```python
from build123d import *

# Parameters (mm, degrees)
SKETCH1_R               = 11.7
BOSS_EXTRUDE1_DEPTH     = 35
SKETCH2_R               = 10
BOSS_EXTRUDE3_DEPTH     = 51.8
SKETCH3_R               = 3
CUT_EXTRUDE1_DEPTH      = 90.32860684
CUT_EXTRUDE1_DEPTH_BACK = 90.32860684
SKETCH6_W               = 28.4
SKETCH6_H               = 118.8
CUT_EXTRUDE3_DEPTH      = 75.564871086
SKETCH8_R               = 10
SKETCH8_R_2             = 3
CUT_EXTRUDE4_DEPTH      = 5
SKETCH7_R               = 4
SKETCH7_R_2             = 3
BOSS_EXTRUDE4_DEPTH     = 5
FILLET1_R               = 10


with BuildPart() as part:
    # Sketch1 → Boss-Extrude1 (new body)
    with BuildSketch(Plane(origin=(0, 0, 0), x_dir=(0, 0, -1), z_dir=(1, 0, 0))):
        Polygon((-28.4, -59.4), (-23.4, -59.4), (-23.4, -14.4), (23.4, -14.4), (23.4, -59.4), (28.4, -59.4), (28.4, 59.4), (-28.4, 59.4), align=None)
        with Locations((0, 24)):
            Circle(SKETCH1_R, mode=Mode.SUBTRACT)
    extrude(amount=BOSS_EXTRUDE1_DEPTH)

    # Sketch2 → Boss-Extrude3 (add)
    with BuildSketch(Plane.XY.offset(28.4)):
        with Locations(Location((17.5, -34.4, 0), (0, 0, 90))):
            Circle(SKETCH2_R)
        with BuildLine():
            Line((0, -24.717541634), (0, -13.4))
            Line((0, -13.4), (35, -13.4))
            Line((35, -13.4), (35, -24.717541634))
            ThreePointArc((35, -24.717541634), (17.5, -14.4), (0, -24.717541634))
        make_face()
    extrude(amount=-BOSS_EXTRUDE3_DEPTH)

    # Sketch3 → Cut-Extrude1 (cut, two sides)
    with BuildSketch(Plane.XY.offset(28.4)) as cut_extrude1_sk:
        with Locations((10.25, 49.4)):
            Circle(SKETCH3_R)
        with Locations((17.5, -34.4)):
            Circle(SKETCH3_R)
        with Locations((10.25, 2.3)):
            Circle(SKETCH3_R)
        with Locations((24.75, 2.3)):
            Circle(SKETCH3_R)
        with Locations((24.75, 49.4)):
            Circle(SKETCH3_R)
    extrude(amount=CUT_EXTRUDE1_DEPTH, mode=Mode.SUBTRACT)
    extrude(cut_extrude1_sk.sketch, amount=-CUT_EXTRUDE1_DEPTH_BACK, mode=Mode.SUBTRACT)

    # Sketch6 → Cut-Extrude3 (cut, through all)
    with BuildSketch(Plane(origin=(35, 0, 0), x_dir=(0, 0, -1), z_dir=(1, 0, 0))):
        with Locations((14.2, 0)):
            Rectangle(SKETCH6_W, SKETCH6_H)
    extrude(amount=-CUT_EXTRUDE3_DEPTH, mode=Mode.SUBTRACT)

    # Sketch8 → Cut-Extrude4 (cut)
    with BuildSketch(Plane(origin=(0, 0, 0), x_dir=(-1, 0, 0), z_dir=(0, 0, -1))):
        with Locations(Location((-17.5, -34.4, 0), (0, 0, 270))):
            Circle(SKETCH8_R)
        with Locations(Location((-17.5, -34.4, 0), (0, 0, 180))):
            Circle(SKETCH8_R_2, mode=Mode.SUBTRACT)
    extrude(amount=-CUT_EXTRUDE4_DEPTH, mode=Mode.SUBTRACT)

    # Sketch7 → Boss-Extrude4 (add)
    with BuildSketch(Plane(origin=(0, 0, 0), x_dir=(-1, 0, 0), z_dir=(0, 0, -1))):
        with Locations(Location((-24.75, 49.4, 0), (0, 0, 270))):
            Circle(SKETCH7_R)
        with Locations(Location((-24.75, 49.4, 0), (0, 0, 180))):
            Circle(SKETCH7_R_2, mode=Mode.SUBTRACT)
        with Locations(Location((-10.25, 49.4, 0), (0, 0, 270))):
            Circle(SKETCH7_R)
        with Locations(Location((-10.25, 49.4, 0), (0, 0, 180))):
            Circle(SKETCH7_R_2, mode=Mode.SUBTRACT)
        with Locations(Location((-24.75, 2.3, 0), (0, 0, 270))):
            Circle(SKETCH7_R)
        with Locations(Location((-24.75, 2.3, 0), (0, 0, 180))):
            Circle(SKETCH7_R_2, mode=Mode.SUBTRACT)
        with Locations(Location((-10.25, 2.3, 0), (0, 0, 270))):
            Circle(SKETCH7_R)
        with Locations(Location((-10.25, 2.3, 0), (0, 0, 180))):
            Circle(SKETCH7_R_2, mode=Mode.SUBTRACT)
    extrude(amount=BOSS_EXTRUDE4_DEPTH)

    # Fillet1
    fillet1_edges = [part.edges().sort_by_distance(p)[0] for p in [
        (0, 59.4, 14.2),
        (35, 59.4, 14.2),
    ]]
    fillet(fillet1_edges, radius=FILLET1_R)


solid = part.part
```
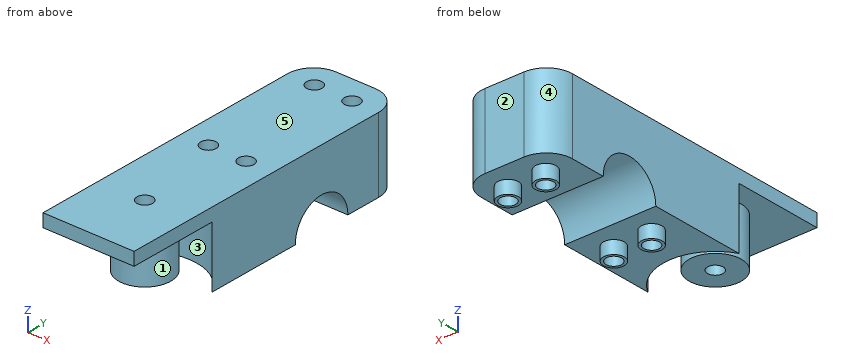
Can you work these out from the model? Positions are in its coordinate system, mm. Face numbers are marked on the shaded views. A direction names the side the tool comes from. Round coordinates to 2 decimals unless told otherwise and drop trailing zeros. Loops run counter-clockwise (first coordinate to the right, second up) from the corner with the lowest first, then second, coordinate; pieces in that order, holes last. Notation, with made-up numbers: M 85.25,-32.5 L 136.25,-32.5 A21 cw 136.25,-25.5 Z; hole C 12,-39.5 d4. An arc over 180 degrees is marked long. Answer in a Markdown table with one row per item.
1. If we section it at C-C, the plane x = 17.5: Please give me the cut outline in (y, z).
Established:
| item | result |
|---|---|
| outline | M -59.4,23.4 L -44.4,23.4 L -44.4,5 L -37.4,5 L -37.4,28.4 L -59.4,28.4 Z; M -31.4,5 L -24.4,5 L -24.4,23.4 L -14.4,23.4 L -14.4,0 L 12.3,0 A11.7 cw 35.7,0 L 59.4,0 L 59.4,28.4 L -31.4,28.4 Z |
2. I'm going to push flat-ended pins straight in: pin 1 Ø10.5 at (x, y) = (19, -41.5) entering from -Z; pin 2 Ø12 at (x, z) = (10.5, 17) entering from -Y; pin 3 Ø5.5 at (x, y) = (10.25, 2.3) entering from -Z; pin 4 Ø3 at (y, z) = (-38.5, 11) entering from -X. Where does each tip first touch, or does it pass through?
Established:
| item | result |
|---|---|
| pin 1 | z = 5 |
| pin 2 | y = -44.35 |
| pin 3 | through |
| pin 4 | x = 7.84 |
3. If we section it at B-B, the plane y = 2.3: Please give me the cut outline in (x, z), plus the area to 3 significant figures.
Established:
| item | result |
|---|---|
| outline | M 0,0 L 6.25,0 L 6.25,-5 L 7.25,-5 L 7.25,28.4 L 0,28.4 Z; M 13.25,-5 L 14.25,-5 L 14.25,0 L 20.75,0 L 20.75,-5 L 21.75,-5 L 21.75,28.4 L 13.25,28.4 Z; M 27.75,-5 L 28.75,-5 L 28.75,0 L 35,0 L 35,28.4 L 27.75,28.4 Z |
| area | 673 mm² |
4. On a 3-axis mill with a long thin cutter (end or side, diameter ignored), from which of +Z, -Z, +X, -X, +Y, -Y can I reach the whole of each face in a straight line? I mean the marked faces 1 and 2. Say none if no direction works.
Established:
| item | result |
|---|---|
| face 1 | -Z |
| face 2 | +Z, -Z, +X, -X, +Y |
5. If we section it at D-D, the plane z = 10: Please give me the cut outline in (x, y).
Established:
| item | result |
|---|---|
| outline | M 0,-24.72 A20 cw 35,-24.72 L 35,17.93 L 0,17.93 Z; M 0,30.07 L 35,30.07 L 35,49.4 A10 ccw 25,59.4 L 10,59.4 A10 ccw 0,49.4 Z; C 17.5,-34.4 d20; hole C 10.25,2.3 d6; hole C 10.25,49.4 d6; hole C 17.5,-34.4 d6; hole C 24.75,2.3 d6; hole C 24.75,49.4 d6 |
6. Thinking about a two-plate mould opening in X: for the marked faces 3, 4 and 5, which applies, pulls with the +X half, pulls with the -X half, needs draft (parallel to the pull), parting line crosses it, or undercut?
Established:
| item | result |
|---|---|
| face 3 | undercut |
| face 4 | pulls with the -X half |
| face 5 | needs draft |
7. Please list where these lines run through material, in increasing order: line 1 (X direction, y = 2, z = 19); line 2 (Y direction, x = 10.25, z = -3.45); line 3 (Y direction, x = 9.5, z = 9). Write a range as from..to.
Established:
| item | result |
|---|---|
| line 1 | 0..7.27, 13.23..21.77, 27.73..35 |
| line 2 | -1.7..-0.7, 5.3..6.3, 45.4..46.4, 52.4..53.4 |
| line 3 | -40.4..-28.4, -16.07..-0.6, 5.2..16.52, 31.48..46.5, 52.3..59.39 |
8. If we section it at A-A, the plane z = 14.5: Please give me the cut outline in (x, y), plus the area to 3 significant figures.
Established:
| item | result |
|---|---|
| outline | M 0,-24.72 A20 cw 35,-24.72 L 35,49.4 A10 ccw 25,59.4 L 10,59.4 A10 ccw 0,49.4 Z; C 17.5,-34.4 d20; hole C 10.25,2.3 d6; hole C 10.25,49.4 d6; hole C 17.5,-34.4 d6; hole C 24.75,2.3 d6; hole C 24.75,49.4 d6 |
| area | 2,820 mm² |
